Geometry check sheet. Reference: the model listing, model coordinates, mm. A direction names the side the tool comes from. Give positions to 0.01 mm unless a question says otherwise; leave off trailing zeros. Loops run counter-clockwise (first coordinate to the right, second up) from the corner with the lowest first, then second, coordinate; pieces in that order, holes last. Notation, with made-up numbers: (6, 79.5) -> (36, 79.5) arc R20 cw to (36, 84.5) -> close; hole circle Ø6 at (18.5, 62). An arc over 180 degrees is marked (long way). Write item = value, one per line. Start each with the question number.
Autodesk Inventor part; units mm, degrees
ref_plane "YZ Plane" through (0, 0, 0) normal (1, 0, 0) x (0, 1, 0)
ref_plane "XZ Plane" through (0, 0, 0) normal (0, 1, 0) x (-1, 0, 0)
ref_plane "XY Plane" through (0, 0, 0) normal (0, 0, 1) x (1, 0, 0)
sketch "Sketch1" plane through (0, 0, 0) normal (0, 1, 0) x (-1, 0, 0)
  line L0 (0, 0) -> (38.1, 0)
  line L1 (38.1, 0) -> (38.1, -88.9)
  line L2 (38.1, -88.9) -> (0, -88.9)
  line L3 (0, -25.4) -> (12.7, -25.4)
  line L4 (12.7, -25.4) -> (12.7, -63.5)
  line L5 (12.7, -63.5) -> (0, -63.5)
  line L6 (0, -88.9) -> (0, -63.5)
  line L7 (0, -25.4) -> (0, 0)
  line L8 (38.1, 0) -> (34.925, 0)
  line L9 (34.925, 0) -> (34.925, -88.9)
  line L10 (34.925, -88.9) -> (38.1, -88.9)
  line L11 (38.1, -88.9) -> (38.1, 0)
  point P0 (12.7, -12.7)
  point P1 (22.225, -31.75)
  point P2 (22.225, -57.15)
  point P3 (12.7, -76.2)
  dimension "d0" = 38.1
  dimension "d1" = 88.9
  dimension "d3" = 38.1
  dimension "d4" = 25.4
  dimension "d5" = 12.7
  dimension "d6" = 12.7
  dimension "d7" = 12.7
  dimension "d8" = 12.7
  dimension "d9" = 15.875
  dimension "d10" = 15.875
  dimension "d11" = 31.75
  dimension "d12" = 31.75
  dimension "d13" = 3.175
  dimension "d35" = 12.7
extrude "Extrusion1" add sketch "Sketch1" along normal blind 3.175
hole "Hole1" at (-12.7, 0, -12.7) at (-22.225, 0, -31.75) at (-22.225, 0, -57.15) at (-12.7, 0, -76.2) direction (0, 1, 0) diameter 6.35 depth 3.175 countersink diameter 9.1948 countersink angle 82
extrude "Extrusion2" add sketch "Sketch1" along normal blind 22.225 and the other way blind 19.05 contours L0 L1 L2 L9
thread "Thread1"
thread "Thread2"
thread "Thread3"
thread "Thread4"
properties part number "t 2 piece" material "Aluminum 6061"
1) Depth check by flat-ended pin: pin 1 Ø10 at (x, z) = (-12.7, -12.7) entering from -Y; pin 2 Ø1.5 at (y, z) = (-14.5, -59) entering from +X (3 decimals); pin 3 Ø7.5 at (x, z) = (-12.7, -76.2) entering from -Y. Enter the tip coordinate at first touch or a pass-through.
2) Section check B-B (x = -33.5). Enter the section's corners in (y, z) (3 decimals), plus the area to 3 significant figures.
3) Section check A-A (z = -12.7). Enter the section's corners in (x, y) (3 decimals), plus the area to 3 significant figures.
4) Thickness scan on line 1 (X direction, y = 2.5, z = -31.75); line 2 (Y direction, x = -2.5, z = -84.5) (3 decimals); line 3 (X direction, y = -7.5, z = -45) (3 decimals). Record the ranges inside material, lowest first.
5) Section check C-C (x = -24). Give the number of separate pieces and of enclosed holes in the cut face, plus the area to 3 significant figures.
6) Tool access check on faces 1 (the flat face through (-17, 3.175, -44)), 2 (the flat face through (0, 2, -76)), 3 (the flat face through (-36, -19.05, -44)), 4 (the flat face through (-34.925, -10, -44)), 5 (the flat face through (-6, 2, -63.5)). Record the directions out of +Z, -Z, +X, -X, +Y, -Y that give a thin tool (end or side, any length) a straight path to the whole face; none if there is none.
7) Section check D-D (y = 20.5). Enter the section's corners in (x, z) (3 decimals), plus the area to 3 significant figures.
Check result:
q1.pin_1 = 0
q1.pin_2 = -34.925
q1.pin_3 = 0.97
q2.outline = (0, -88.9) -> (3.175, -88.9) -> (3.175, 0) -> (0, 0) -> close
q2.area = 282 mm2
q3.outline = (-38.1, -19.05) -> (-34.925, -19.05) -> (-34.925, 0) -> (-17.297, 0) -> (-15.875, 1.636) -> (-15.875, 3.175) -> (-34.925, 3.175) -> (-34.925, 22.225) -> (-38.1, 22.225) -> close; (-9.525, 1.636) -> (-8.103, 0) -> (0, 0) -> (0, 3.175) -> (-9.525, 3.175) -> close
q3.area = 219 mm2
q4.line_1 = -38.1 to -25.4, -19.05 to -12.7
q4.line_2 = 0 to 3.175
q4.line_3 = -38.1 to -34.925
q5.separate_pieces = 3
q5.enclosed_holes = 0
q5.area = 243 mm2
q6.face_1 = +Z, -Z, +X, +Y
q6.face_2 = +Z, -Z, +X, +Y, -Y
q6.face_3 = +Z, -Z, +X, -X, -Y
q6.face_4 = +Z, -Z, +X, -Y
q6.face_5 = +X, +Y, -Y
q7.outline = (-38.1, -88.9) -> (-34.925, -88.9) -> (-34.925, 0) -> (-38.1, 0) -> close
q7.area = 282 mm2
